```python
from build123d import *

# Parameters (mm, degrees)
SKETCH1_R           = 35
BOSS_EXTRUDE1_DEPTH = 3
BOSS_EXTRUDE2_START = 6
BOSS_EXTRUDE2_DEPTH = 6
BOSS_EXTRUDE3_DEPTH = 6


with BuildPart() as part:
    # Sketch1 → Boss-Extrude1 (new, symmetric)
    with BuildSketch(Plane.XY):
        Circle(SKETCH1_R)
    extrude(amount=BOSS_EXTRUDE1_DEPTH, both=True)

    # Sketch2 → Boss-Extrude2 (add)
    with BuildSketch(Plane.XY.offset(3).offset(BOSS_EXTRUDE2_START)):
        with BuildLine():
            Line((34.641016151, 5), (-34.641016151, 5))
            ThreePointArc((-34.641016151, 5), (-35, 0), (-34.641016151, -5))
            Line((-34.641016151, -5), (34.641016151, -5))
            ThreePointArc((34.641016151, -5), (35, 0), (34.641016151, 5))
        make_face()
    extrude(amount=-BOSS_EXTRUDE2_DEPTH)

    # Sketch3 → Boss-Extrude3 (add)
    with BuildSketch(Plane(origin=(0, 0, -3), x_dir=(-1, 0, 0), z_dir=(0, 0, -1))):
        with BuildLine():
            Line((5, -34.641016151), (5, 34.641016151))
            ThreePointArc((5, 34.641016151), (0, 35), (-5, 34.641016151))
            Line((-5, 34.641016151), (-5, -34.641016151))
            ThreePointArc((-5, -34.641016151), (0, -35), (5, -34.641016151))
        make_face()
    extrude(amount=BOSS_EXTRUDE3_DEPTH)


solid = part.part
```
Check sheet for the modelled part. Datum: model origin and axes. Units: mm. A direction names the side the tool comes from. Give positions to 0.01 mm unless a question says otherwise; leave off trailing zeros. Write each loop counter-clockwise with the first axis right and the second up, starting at its lowest first coordinate (ties: lowest second). Pieces come first, ordered by that corner, then holes.
Item 1: Cross-section at C-C (z = 7.75). Enter the section's corners in (x, y), and give its area (3 significant figures).
Item 2: Access from +Z, -Z, +X, -X, +Y, -Y to the whole of each face (thin tool, end or side, straight path). Record for faces 1 (the face through (-5, 0, -6)), 2 (the face through (5, 0, -6)), 3 (the face through (0, 5, 6)).
Item 3: Cross-section at B-B (x = -28). Enter the section's corners in (y, z), and give its area (3 significant figures).
Item 4: Cross-section at D-D (x = 0). Enter the section's corners in (y, z).
Item 5: Gauge pin test, flat ends, axial feed: pin 1 (3 mm diameter, centred on x = -5, z = -3, fed in from +Y); pin 2 (15 mm diameter, centred on x = 19.5, y = -2, fed in from -Z); pin 3 (6 mm diameter, centred on x = 18, z = -1, fed in from -Y). Record the tip position at first contact, or that the pin passes through.
Item 6: Scan lines: L1, parallel to Y at x = -8, z = 4; L2, parallel to Z at x = 25, y = -2; L3, parallel to Z at x = -20, y = 9.5. Record each from-to range of solid material in increasing order.
Item 7: Cross-section at A-A (y = 0). Enter the section's corners in (x, z), and give its area (3 significant figures).
Report:
1. outline: (-34.64, -5) - (34.64, -5) arc R35 ccw to (34.64, 5) - (-34.64, 5) arc R35 ccw to start
1. area: 698 mm2
2. face 1: -Z, -X, +Y, -Y
2. face 2: -Z, +X, +Y, -Y
2. face 3: +Z, +X, -X, +Y
3. outline: (-21, -3) - (21, -3) - (21, 3) - (5, 3) - (5, 9) - (-5, 9) - (-5, 3) - (-21, 3) - close
3. area: 312 mm2
4. outline: (-35, -9) - (35, -9) - (35, 3) - (5, 3) - (5, 9) - (-5, 9) - (-5, 3) - (-35, 3) - close
5. pin 1: stops at y = 34.82
5. pin 2: stops at z = -3
5. pin 3: stops at y = -31.62
6. L1: y = -5 to 5
6. L2: z = -3 to 9
6. L3: z = -3 to 3
7. outline: (-35, -3) - (-5, -3) - (-5, -9) - (5, -9) - (5, -3) - (35, -3) - (35, 9) - (-35, 9) - close
7. area: 900 mm2
